Build history of the part. All positions in model axes, mm. A direction names the side the tool comes from. Round coordinates to 2 decimals unless told otherwise and drop trailing zeros. Loops run counter-clockwise (first coordinate to the right, second up) from the corner with the lowest first, then second, coordinate; pieces in that order, holes last. Notation, with made-up numbers: (-28, -24.5) -> (-15, -24.5) arc R20 cw to (-15, -11.5) -> close; hole circle Ø8 at (-37.75, 33.5). An arc over 180 degrees is marked (long way). Put each result on its own line as item: value. Start each with the question number.
Item 1: Pull direction Z, two halves, no side cores. Call faces 1 (the flat face through (-17, 3, -5)), 2 (the flat face through (0, 5, 0)), 3 (the cylindrical face through (-0.56, 2.54, 12.54)), 4 (the cylindrical face through (-11.273, 2.535, 24.493)): +Z half, -Z half, draft (parallel to the pull), parting line (faces both ways), or undercut.
Item 2: Cut at D-D, the plane x = 15. List the corners of the cut face in (y, z), plus the area to 3 significant figures.
Item 3: Cut at A-A, the plane x = 1. List the corners of the cut face in (y, z), plus the area to 3 significant figures.
Item 4: Cut at C-C, the plane y = 2.4. List the corners of the cut face in (x, z) (3 decimals).
Item 5: Tool access for faces 5 (the flat face through (-14.125, 2, -16)), 6 (the flat face through (0, 2, 27.5)), 7 (the flat face through (14.125, 2, -16)), 8 (the flat face through (-17, 3, 5)), 9 (the flat face through (14.125, 2, 11)): list every direction of +Z, -Z, +X, -X, +Y, -Y with a clear straight run to the whole face (end or side of a thin tool).
Item 6: Drill centre lines: probe 1 along X at (y, z) = (3.25, 10) (3 decimals); probe 2 along Z at (x, y) = (0, 2.5); probe 3 along X at (y, z) = (0.45, -13) (3 decimals). Where is each one in solid material? Low to high. Write a range as [from, to].
Item 7: Cut at B-B, the plane z = 10. List the corners of the cut face in (x, y) (3 decimals), plus the area to 3 significant figures.
Item 8: Flat gauge pins, fed straight in: pin 1 Ø1.5 at (y, z) = (2, 11.5) entering from +X (3 decimals); pin 2 Ø2.5 at (x, y) = (17.5, 3) entering from -Z; pin 3 Ø1.5 at (x, y) = (-18, 3) entering from +Z. Where does each tip first touch, or does it go through?
```python
from build123d import *

# Parameters (mm, degrees)
SKETCH1_W           = 28.25
SKETCH1_H           = 55
BOSS_EXTRUDE1_DEPTH = 5
SKETCH3_W           = 5.9
SKETCH3_H           = 10
BOSS_EXTRUDE2_DEPTH = 5
SKETCH2_R           = 2.6
CUT_EXTRUDE1_DEPTH  = 10
FILLET1_R           = 10


with BuildPart() as part:
    # Sketch1 → Boss-Extrude1 (new body)
    with BuildSketch(Plane(origin=(0, 0, 0), x_dir=(1, 0, 0), z_dir=(0, 1, 0))):
        Rectangle(SKETCH1_W, SKETCH1_H)
    extrude(amount=BOSS_EXTRUDE1_DEPTH)

    # Sketch3 → Boss-Extrude2 (add)
    with BuildSketch(Plane(origin=(0, 5, 0), x_dir=(1, 0, 0), z_dir=(0, 1, 0))):
        with Locations((-17.075, 0)):
            Rectangle(SKETCH3_W, SKETCH3_H)
        with Locations((17.075, 0)):
            Rectangle(SKETCH3_W, SKETCH3_H)
    extrude(amount=-BOSS_EXTRUDE2_DEPTH)

    # Sketch2 → Cut-Extrude1 (cut)
    with BuildSketch(Plane(origin=(0, 5, 0), x_dir=(1, 0, 0), z_dir=(0, 1, 0))):
        with Locations((0, -10)):
            Circle(SKETCH2_R)
    extrude(amount=-CUT_EXTRUDE1_DEPTH, mode=Mode.SUBTRACT)

    # Fillet1
    fillet1_edges = [part.edges().sort_by_distance(p)[0] for p in [
        (14.125, 2.5, 27.5),
        (-14.125, 2.5, 27.5),
    ]]
    fillet(fillet1_edges, radius=FILLET1_R)


solid = part.part
```
Reply:
1. face 1: -Z half
1. face 2: draft
1. face 3: undercut
1. face 4: +Z half
2. outline: (0, -5) -> (5, -5) -> (5, 5) -> (0, 5) -> close
2. area: 50.0 mm^2
3. outline: (0, -27.5) -> (5, -27.5) -> (5, 7.6) -> (0, 7.6) -> close; (0, 12.4) -> (5, 12.4) -> (5, 27.5) -> (0, 27.5) -> close
3. area: 251 mm^2
4. outline: (-20.025, -5) -> (-14.125, -5) -> (-14.125, -27.5) -> (14.125, -27.5) -> (14.125, -5) -> (20.025, -5) -> (20.025, 5) -> (14.125, 5) -> (14.125, 17.5) arc R10 ccw to (4.125, 27.5) -> (-4.125, 27.5) arc R10 ccw to (-14.125, 17.5) -> (-14.125, 5) -> (-20.025, 5) -> close; hole circle Ø5.2 at (0, 10)
5. face 5: -Z, -X, +Y, -Y
5. face 6: +Z, +X, -X, +Y, -Y
5. face 7: -Z, +X, +Y, -Y
5. face 8: +Z, -X, +Y, -Y
5. face 9: +Z, +X, +Y, -Y
6. probe 1: x = [-14.125, -2.6], [2.6, 14.125]
6. probe 2: z = [-27.5, 7.4], [12.6, 27.5]
6. probe 3: x = [-14.125, 14.125]
7. outline: (-14.125, 0) -> (-2.6, 0) -> (-2.6, 5) -> (-14.125, 5) -> close; (2.6, 0) -> (14.125, 0) -> (14.125, 5) -> (2.6, 5) -> close
7. area: 115 mm^2
8. pin 1: stops at x = 14.125
8. pin 2: stops at z = -5
8. pin 3: stops at z = 5
